Source: CAD feature listing. Evaluate the final solid. Frame: model axes, mm. Give positions to 0.01 mm unless a question says otherwise; leave off trailing zeros. Write each loop counter-clockwise with the first axis right and the second up, starting at its lowest first coordinate (ties: lowest second). Pieces come first, ordered by that corner, then holes. Notation, with made-up numbers: (-14.75, 47.5) - (44.25, 47.5) arc R23 ccw to (44.25, 81.5) - close; hole circle Ø1 at (-36.5, -6.75). An arc over 180 degrees is marked (long way). Answer as a JSON object with one key per item and string values. Group by question number.
from build123d import *

# Parameters (mm, degrees)
SKETCH1_R           = 1.5
BOSS_EXTRUDE1_DEPTH = 3


with BuildPart() as part:
    # Sketch1 → Boss-Extrude1 (new body)
    with BuildSketch(Plane(origin=(0, 0, 0), x_dir=(1, 0, 0), z_dir=(0, 1, 0))):
        with BuildLine():
            ThreePointArc((10.653057646, -20.439235866), (10.054560804, -24.397448123), (6.743799383, -26.647892869))
            Line((6.743799383, -26.647892869), (6.743799383, -43.647892869))
            ThreePointArc((6.743799383, -43.647892869), (11.280986361, -53.065151094), (0.993799383, -54.921115062))
            Line((0.993799383, -54.921115062), (0.993799383, -43.647892869))
            Line((0.993799383, -43.647892869), (0.993799383, -23.027426317))
            Line((0.993799383, -23.027426317), (-4.829629131, -1.294095226))
            ThreePointArc((-4.829629131, -1.294095226), (-1.294095226, 4.829629131), (4.829629131, 1.294095226))
            Line((4.829629131, 1.294095226), (10.653057646, -20.439235866))
        make_face()
        with Locations(Location((5.823428515, -21.733331092, 0), (0, 0, 270))):
            Circle(SKETCH1_R, mode=Mode.SUBTRACT)
        with Locations(Location((0, 0, 0), (0, 0, 270))):
            Circle(SKETCH1_R, mode=Mode.SUBTRACT)
    extrude(amount=BOSS_EXTRUDE1_DEPTH)


solid = part.part
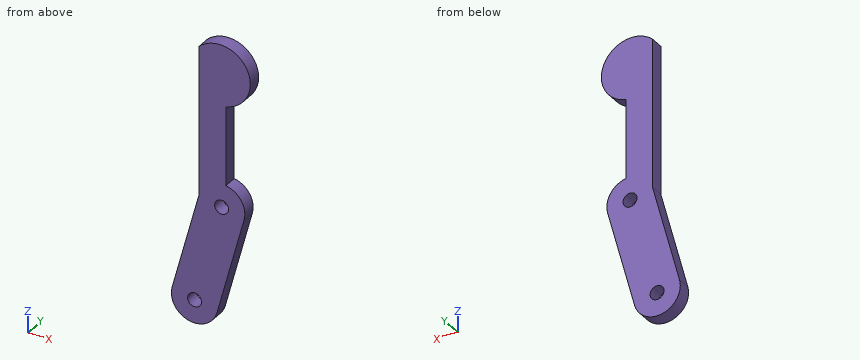
Q1. Section B-B on z = 0. Return the cut outline in (x, y).
Q2. Section A-A on x = 9. Return the cut outline in (y, z).
Q3. Section C-C on y = 2.1. Return the cut outline in (x, z), then the cut area to 3 significant figures.
Q4. First-contact query: pin 1 Ø1 at (y, z) = (2.5, 27.5) entering from -X; pin 2 Ø0.9 at (y, z) = (2, 36.5) entering from +X; pin 3 Ø1 at (y, z) = (0.5, 6) entering from -X. Flat tips, straight axial feed; report the tip coordinate or a pass-through.
Q5. Ray query, probe 1 along X at (y, z) = (1.45, 27); probe 2 along X at (y, z) = (2.15, 23); probe 3 along X at (y, z) = (1.4, 0). Return the intervals inside material, ascending. Write a range as [from, to].
Q6. Section D-D on z = 47. Return the cut outline in (x, y).
Taken from the geometry:
{
 "1": {"outline": "(-5, 0) - (-1.5, 0) - (-1.5, 3) - (-5, 3) - close; (1.5, 0) - (5.18, 0) - (5.18, 3) - (1.5, 3) - close"},
 "2": {"outline": "(0, 14.27) - (3, 14.27) - (3, 25.59) - (0, 25.59) - close; (0, 44.57) - (3, 44.57) - (3, 55.59) - (0, 55.59) - close"},
 "3": {"outline": "(-4.83, 1.29) arc R5 ccw to (4.83, -1.29) - (10.65, 20.44) arc R5 ccw to (6.74, 26.65) - (6.74, 43.65) arc R6.57 ccw (long way) to (0.99, 54.92) - (0.99, 23.03) - close; hole circle Ø3 at (0, 0); hole circle Ø3 at (5.82, 21.73)", "area": "514 mm²"},
 "4": {"pin 1": "stops at x = 0.99", "pin 2": "stops at x = 6.74", "pin 3": "stops at x = -3.7"},
 "5": {"probe 1": "x = [0.99, 6.74]", "probe 2": "x = [0.99, 5.02], [6.63, 10.66]", "probe 3": "x = [-5, -1.5], [1.5, 5.18]"},
 "6": {"outline": "(0.99, 0) - (11.23, 0) - (11.23, 3) - (0.99, 3) - close"}
}
